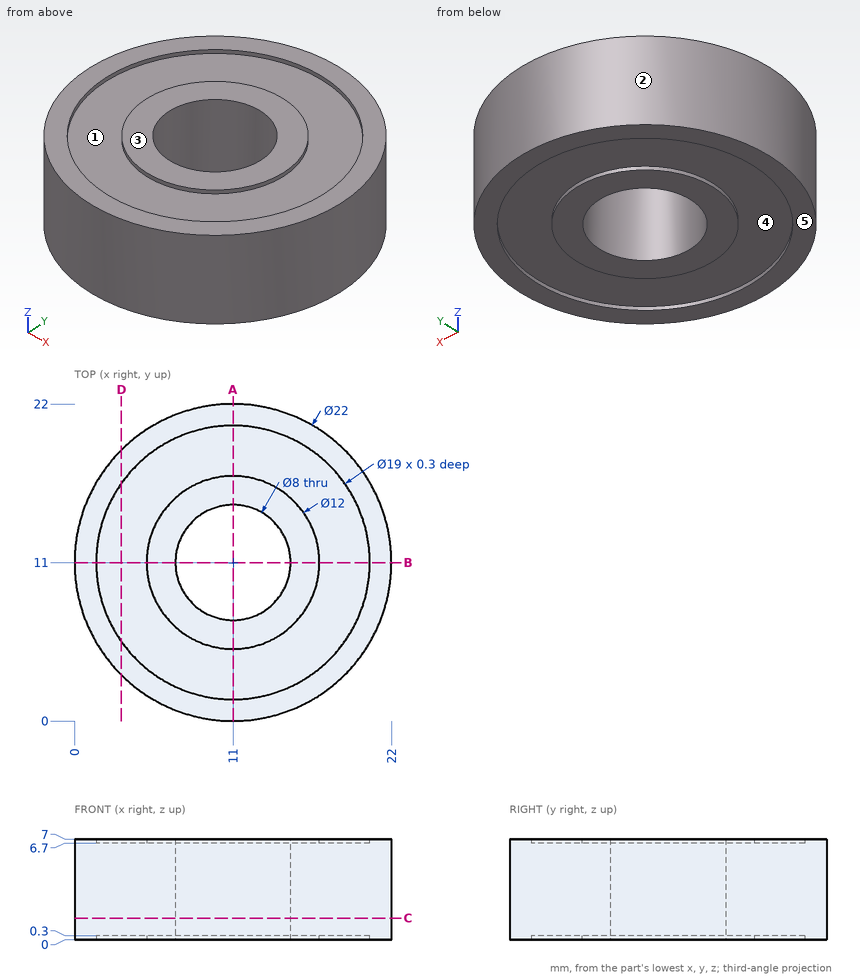
Verification items for this drawing (mm, ordinates from the low corner). A direction names the side the tool comes from. Give positions to 0.01 mm unless a question says otherwise; leave off trailing zeros. Loops run counter-clockwise (first coordinate to the right, second up) from the corner with the lowest first, then second, coordinate; pieces in that order, holes last. Notation, with made-up numbers: (44.5, 15.25) - (57.5, 15.25) arc R16 cw to (57.5, 39.25) - close; hole circle Ø11 at (-0.75, 84.25). An arc over 180 degrees is marked (long way). Write item = value, one per line. Start each with the question number.
Q1. Cross-section at D-D, the plane x = 3.25. Enter the section's corners in (y, z), and give its area (3 significant figures).
Q2. Mould release check, pull along Y, two halves, no side actions. Record for the marked faces 1, 2 and 3: released by +Y, released by -Y, zero draft, split by the parting line, or undercut.
Q3. Depth check by flat-ended pin: P1, Ø2, axis at y = 14.5, z = 4, coming from the -X side; P2, Ø1, axis at y = 13, z = 2, coming from the +X side; P3, Ø7, axis at x = 11, y = 11, coming from the -Z side; P4, Ø3, axis at y = 3.5, z = 4.5, coming from the -X side. Enter the tip coordinate at first touch or a pass-through.
Q4. Tool access check on the marked faces 4 and 5. Record the directions out of +Z, -Z, +X, -X, +Y, -Y that give a thin tool (end or side, any length) a straight path to the whole face; none if there is none.
Q5. Thickness scan on line 1 (Y direction, x = 11, z = 6.95); line 2 (X direction, y = 11.5, z = 6.75); line 3 (Y direction, x = 11, z = 0.75). Record the ranges inside material, lowest first.
Q6. Cross-section at A-A, the plane x = 11. Enter the section's corners in (y, z).
Q7. Cross-section at C-C, the plane z = 1.5. Enter the section's corners in (x, y), and give its area (3 significant figures).
Answer key:
q1.outline = (3.19, 0) - (5.51, 0) - (5.51, 0.3) - (16.49, 0.3) - (16.49, 0) - (18.81, 0) - (18.81, 7) - (16.49, 7) - (16.49, 6.7) - (5.51, 6.7) - (5.51, 7) - (3.19, 7) - close
q1.area = 103 mm^2
q2.face_1 = undercut
q2.face_2 = split by the parting line
q2.face_3 = zero draft
q3.P1 = 0.29
q3.P2 = 21.9
q3.P3 = through
q3.P4 = 1.78
q4.face_4 = -Z
q4.face_5 = -Z, +X, -X, +Y, -Y
q5.line_1 = 0 to 1.5, 5 to 7, 15 to 17, 20.5 to 22
q5.line_2 = 0.01 to 1.51, 5.02 to 7.03, 14.97 to 16.98, 20.49 to 21.99
q5.line_3 = 0 to 7, 15 to 22
q6.outline = (0, 0) - (1.5, 0) - (1.5, 0.3) - (5, 0.3) - (5, 0) - (7, 0) - (7, 7) - (5, 7) - (5, 6.7) - (1.5, 6.7) - (1.5, 7) - (0, 7) - close; (15, 0) - (17, 0) - (17, 0.3) - (20.5, 0.3) - (20.5, 0) - (22, 0) - (22, 7) - (20.5, 7) - (20.5, 6.7) - (17, 6.7) - (17, 7) - (15, 7) - close
q7.outline = circle Ø22 at (11, 11); hole circle Ø8 at (11, 11)
q7.area = 330 mm^2
